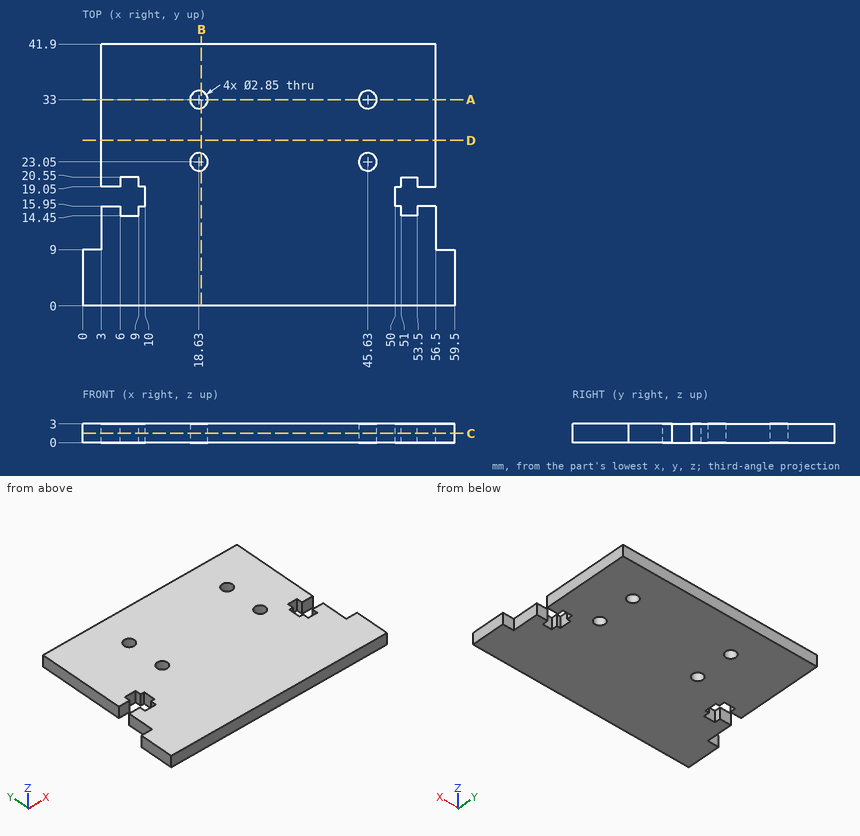
Study the drawing (mm; zero at the part's minimum x, y, z) and answer. Give positions to 0.01 mm unless a question says otherwise; leave off trailing zeros. Write each loop counter-clockwise with the first axis right and the second up, starting at its lowest first coordinate (ties: lowest second). Pieces come first, ordered by that corner, then holes. Notation, with made-up numbers: (23, 62.25) -> (70, 62.25) arc R18 ccw to (70, 70.25) -> close; hole circle Ø1 at (83, 81). An arc over 180 degrees is marked (long way). Write item = value, one per line. Start each with the question number.
1) The part is cut by section B-B, the plane x = 19. Determine the outline of the cut face in (y, z) (1 decimal), and give its area (3 significant figures).
2) Each of these flat-tipped pins is pushed along its axis until it touches: pin 1 (1.5 mm diameter, centred on y = 35, z = 1, fed in from +X); pin 2 (0.9 mm diameter, centred on y = 17, z = 1, fed in from +X); pin 3 (1.6 mm diameter, centred on y = 20, z = 1.5, fed in from -X). Where does it stop, or does it pass through?
3) The part is cut by section C-C, the plane z = 1.5. Count the separate pieces of the cut face and the enclosed holes in it, and give its area (3 significant figures).
4) Straight lines are drawn through the part: line 1 along Y through (x, z) = (4.5, 1); line 2 along Y through (x, z) = (19.5, 1.95); line 3 along X through (y, z) = (14, 1.2). For each, find the intervals that lie inside material, in ascending order.
5) The part is cut by section D-D, the plane y = 26.5. Determine the outline of the cut face in (x, z).
6) The part is cut by section A-A, the plane y = 33. Determine the outline of the cut face in (x, z) (1 decimal).
Solutions:
q1.outline = (0, 0) -> (21.7, 0) -> (21.7, 3) -> (0, 3) -> close; (24.4, 0) -> (31.6, 0) -> (31.6, 3) -> (24.4, 3) -> close; (34.4, 0) -> (41.9, 0) -> (41.9, 3) -> (34.4, 3) -> close
q1.area = 109 mm²
q2.pin_1 = 56.5
q2.pin_2 = 50
q2.pin_3 = 3
q3.separate_pieces = 1
q3.enclosed_holes = 4
q3.area = 2,210 mm²
q4.line_1 = 0 to 15.95, 19.05 to 41.9
q4.line_2 = 0 to 21.92, 24.18 to 31.87, 34.13 to 41.9
q4.line_3 = 3 to 56.5
q5.outline = (3, 0) -> (56.5, 0) -> (56.5, 3) -> (3, 3) -> close
q6.outline = (3, 0) -> (17.2, 0) -> (17.2, 3) -> (3, 3) -> close; (20.1, 0) -> (44.2, 0) -> (44.2, 3) -> (20.1, 3) -> close; (47.1, 0) -> (56.5, 0) -> (56.5, 3) -> (47.1, 3) -> close
